from build123d import *

# Parameters (mm, degrees)
F0_W      = 8.89
F0_H      = 10.922
F1_DEPTH  = 3.302
F3_DEPTH  = 13.462
F4_R      = 0.508
F4_R_2    = 1.6374420612
F5_DEPTH  = 0.3048
F6_R      = 1.6374420612
F7_DEPTH  = 0.254
F8_W      = 8.89
F8_H      = 6.604
F9_DEPTH  = 8.3439
F10_W     = 2.667
F10_H     = 2.4411697693
F11_DEPTH = 0.3048
F12_W     = 2.667
F12_H     = 2.4411697693
F13_DEPTH = 0.6096
F14_R     = 2.75
F15_DEPTH = 5.08
F16_SIZE  = 0.127
F18_R     = 0.508
F19_DEPTH = 0.254
F20_R     = 0.508
F21_DEPTH = 0.3048
F22_R     = 0.254
F23_R     = 1.016
F24_DEPTH = 4.5974
F25_R     = 1.016
F26_R     = 0.508


with BuildPart() as f1:
    # F0 (on Front) → F1 (new body)
    with BuildSketch(Plane.XZ):
        with Locations((0, -1.143)):
            Rectangle(F0_W, F0_H)
    extrude(amount=F1_DEPTH)

    # F2 (on face) → F3 (join)
    with BuildSketch(Plane(origin=(0, 0, 0), x_dir=(-1, 0, 0), z_dir=(0, 1, 0))):
        with BuildLine():
            ThreePointArc((4.191, 0), (0, 4.191), (-4.191, 0))
            Line((-4.191, 0), (-4.191, -6.2759071589))
            Line((-4.191, -6.2759071589), (4.191, -6.2759071589))
            Line((4.191, -6.2759071589), (4.191, 0))
        make_face()
    extrude(amount=-F3_DEPTH)

    # F4 (on face) → F5 (join)
    with BuildSketch(Plane.XZ.offset(13.462)):
        with BuildLine():
            Line((1.524, -9.398), (1.524, -1.3935676202))
            ThreePointArc((1.524, -1.3935676202), (0, 2.0650924222), (-1.524, -1.3935676202))
            Line((-1.524, -1.3935676202), (-1.524, -9.398))
            ThreePointArc((-1.524, -9.398), (-1.0776307345, -10.4756307345), (0, -10.922))
            ThreePointArc((0, -10.922), (1.0776307345, -10.4756307345), (1.524, -9.398))
        make_face()
        with Locations((0, -9.398)):
            Circle(F4_R, mode=Mode.SUBTRACT)
        Circle(F4_R_2, mode=Mode.SUBTRACT)
        Circle(F4_R_2)
    extrude(amount=F5_DEPTH)

    # F6 (on face) → F7 (join)
    with BuildSketch(Plane.XZ.offset(13.7668)):
        Circle(F6_R)
    extrude(amount=F7_DEPTH)

    # F8 (on face) → F9 (join)
    with BuildSketch(Plane.XZ.offset(3.302)):
        with Locations((0, -3.302)):
            Rectangle(F8_W, F8_H)
    extrude(amount=F9_DEPTH)

    # F10 (on face) → F11 (join, through all)
    with BuildSketch(Plane.XZ.offset(13.462)):
        with Locations((-2.8575, -5.0553222742)):
            Rectangle(F10_W, F10_H)
        with Locations((2.8575, -5.0553222742)):
            Rectangle(F10_W, F10_H)
    extrude(amount=F11_DEPTH)

    # F12 (on face) → F13 (join)
    with BuildSketch(Plane.XZ.offset(13.7668)):
        with Locations((-2.8575, -5.0553222742)):
            Rectangle(F12_W, F12_H)
        with Locations((2.8575, -5.0553222742)):
            Rectangle(F12_W, F12_H)
    extrude(amount=F13_DEPTH)

    # F14 (on face) → F15 (cut)
    with BuildSketch(Plane(origin=(0, 0, 0), x_dir=(-1, 0, 0), z_dir=(0, 1, 0))):
        Circle(F14_R)
    extrude(amount=-F15_DEPTH, mode=Mode.SUBTRACT)

    # F16
    f16_edges = [f1.edges().sort_by_distance(p)[0] for p in [
        (-4.445, -1.651, 4.318),
        (4.445, -1.651, 4.318),
        (4.445, -5.82295, -6.604),
        (-4.445, -5.82295, -6.604),
        (2.75, 0, 0),
    ]]
    chamfer(f16_edges, length=F16_SIZE)

    # F18 (on offset) → F19 (join)
    with BuildSketch(Plane.XZ.offset(7.7724)):
        with BuildLine():
            Line((1.27, -6.604), (-1.27, -6.604))
            Line((-1.27, -6.604), (-1.27, -9.652))
            ThreePointArc((-1.27, -9.652), (-0.8980256121, -10.5500256121), (0, -10.922))
            ThreePointArc((0, -10.922), (0.8980256121, -10.5500256121), (1.27, -9.652))
            Line((1.27, -9.652), (1.27, -6.604))
        make_face()
        with Locations((0, -9.398)):
            Circle(F18_R, mode=Mode.SUBTRACT)
    extrude(amount=-F19_DEPTH)

    # F20 (on face) → F21 (join)
    with BuildSketch(Plane(origin=(-4.445, 0, 0), x_dir=(0, -1, 0), z_dir=(-1, 0, 0))):
        with BuildLine():
            Line((11.6459, -3.0857360969), (9.6139, -3.0857360969))
            Line((9.6139, -3.0857360969), (9.6139, -9.906))
            ThreePointArc((9.6139, -9.906), (9.9114795103, -10.6244204897), (10.6299, -10.922))
            ThreePointArc((10.6299, -10.922), (11.3483204897, -10.6244204897), (11.6459, -9.906))
            Line((11.6459, -9.906), (11.6459, -3.0857360969))
        make_face()
        with Locations((10.6299, -9.906)):
            Circle(F20_R, mode=Mode.SUBTRACT)
    extrude(amount=F21_DEPTH)

    # F22
    f22_edges = [f1.edges().sort_by_distance(p)[0] for p in [
        (-4.7498, -10.6299, -3.085736),
    ]]
    fillet(f22_edges, radius=F22_R)

    # F23 (on face) → F24 (join)
    with BuildSketch(Plane(origin=(0, -5.08, 0), x_dir=(-1, 0, 0), z_dir=(0, 1, 0))):
        Circle(F23_R)
    extrude(amount=F24_DEPTH)

    # F25
    f25_edges = [f1.edges().sort_by_distance(p)[0] for p in [
        (1.016, -0.4826, 0),
    ]]
    fillet(f25_edges, radius=F25_R)

    # F26
    f26_edges = [f1.edges().sort_by_distance(p)[0] for p in [
        (-4.445, 0, -1.143),
        (4.445, 0, -1.143),
    ]]
    fillet(f26_edges, radius=F26_R)


solid = f1.part
Read the model definition and answer for the solid it produces. Units are mm, in the model's axes. A direction names the side the tool comes from. Round coordinates to 2 decimals unless told otherwise and drop trailing zeros. Order: outer loops, then holes, each group sorted by start corner. A loop starts at its lowest first (then second) coordinate and runs counter-clockwise, first axis right, second up.
1) The mould has two halves that part along Z. Classify faces 1 (the face through (3, -14.376, -5)), 2 (the face through (-0.09, -8.31, 4.19)), 3 (the face through (-4.595, -11.114, -9.753)): released by +Z, released by -Z, zero draft, split by the parting line, or undercut.
2) The part is cut by section B-B on y = -7.25. Write down the section's boundary in (x, z) (3 decimals).
3) Straight lines are drawn through the part: L1, parallel to Z at x = 0, y = -2.95; L2, parallel to Z at x = 0, y = -3.6; L3, parallel to Z at x = 0, y = -13.65. For each, find the intervals that lie inside material, in ascending order.
4) The part is cut by section C-C on y = -12.5. Write down the section's boundary in (x, z).
5) For faces 4 (the face through (4.191, -13, -3)), 5 (the face through (0.22, -3.31, -0.99)), 6 (the face through (2, -3.302, 4)), 7 (the face through (0.067, -13.612, 2.064)), 8 (the face through (0, -13.462, -8.6)), determine the directions among +Z, -Z, +X, -X, +Y, -Y from which every point of the face is accessible in a straight line to the end or side of a thin tool.
6) The part is cut by section A-A on y = -2.5. Write down the section's boundary in (x, z) (3 decimals).
7) Flat-ended cylindrical pins translate along their axes: pin 1 (1.5 mm diameter, centred on y = -2, z = 0, fed in from -X) (3 decimals); pin 2 (3.5 mm diameter, centred on x = 0.5, z = -9.5, fed in from +Y); pin 3 (1.6 mm diameter, centred on y = -10.63, z = -9.91, fed in from -X); pin 4 (3.5 mm diameter, centred on x = -1, z = 1.5, fed in from -Y). Find the tip coordinate at first contact, or state that the pin passes through.
Resolved:
1. face 1: zero draft
1. face 2: released by +Z
1. face 3: undercut
2. outline: (-4.445, -6.477) - (-4.318, -6.604) - (4.318, -6.604) - (4.445, -6.477) - (4.445, 0) - (4.191, 0) arc R4.191 ccw to (-4.191, 0) - (-4.445, 0) - close
3. L1: z = -6.6 to -2.75, -1.02 to 1.02, 2.75 to 4.32
3. L2: z = -6.6 to -2.75, -1.02 to 1.02, 2.75 to 4.19
3. L3: z = -10.92 to -9.91, -8.89 to 2.07
4. outline: (-4.19, -6.28) - (4.19, -6.28) - (4.19, 0) arc R4.19 ccw to (-4.19, 0) - close
5. face 4: +Z, -Z, +X, -Y
5. face 5: +Y
5. face 6: +Z, -Y
5. face 7: -Y
5. face 8: -Z, +X, -X
6. outline: (-4.445, -6.477) - (-4.318, -6.604) - (4.318, -6.604) - (4.445, -6.477) - (4.445, 4.191) - (4.318, 4.318) - (-4.318, 4.318) - (-4.445, 4.191) - close; circle Ø2.032 at (0, 0); hole circle Ø5.5 at (0, 0)
7. pin 1: stops at x = -4.445
7. pin 2: stops at y = -7.52
7. pin 3: stops at x = -4.75
7. pin 4: stops at y = -14.02
